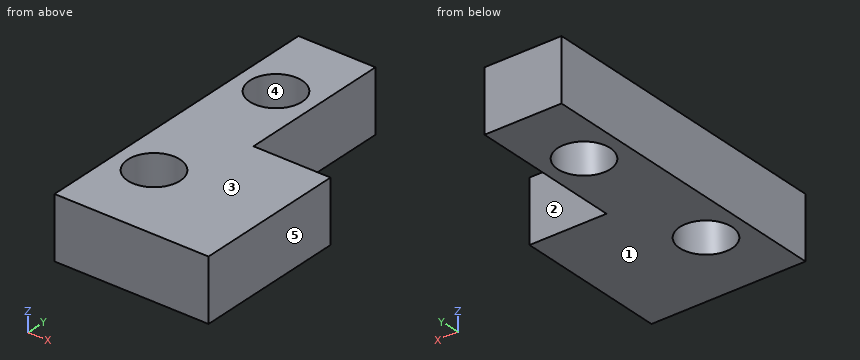
```python
from build123d import *

# Parameters (mm, degrees)
ESQUISSE1_W             = 10
ESQUISSE1_H             = 20
BOSS_EXTRU_1_DEPTH      = 4
D_GAGEMENT_M33_D        = 3.4
ESQUISSE2_W             = 5
ESQUISSE2_H             = 10
ENL_V_MAT_EXTRU_2_DEPTH = 4


with BuildPart() as part:
    # Esquisse1 → Boss.-Extru.1 (new body)
    with BuildSketch(Plane.XY):
        Rectangle(ESQUISSE1_W, ESQUISSE1_H)
    extrude(amount=BOSS_EXTRU_1_DEPTH)

    # Dégagement M33 (through all)
    with Locations(Plane(origin=(0, 0, 0), x_dir=(-1, 0, 0), z_dir=(0, 0, -1))):
        with Locations((2.5, 5), (2.5, -5)):
            Hole(D_GAGEMENT_M33_D / 2)

    # Esquisse2 → Enlèv. mat.-Extru.2 (cut)
    with BuildSketch(Plane(origin=(0, 0, 0), x_dir=(-1, 0, 0), z_dir=(0, 0, -1))):
        with Locations((-2.5, 5)):
            Rectangle(ESQUISSE2_W, ESQUISSE2_H)
    extrude(amount=-ENL_V_MAT_EXTRU_2_DEPTH, mode=Mode.SUBTRACT)


solid = part.part
```
The model under review builds one solid part; all positions refer to its coordinate system, in mm. Face numbers are marked on the shaded views. A direction names the side the tool comes from. Give positions to 0.01 mm unless a question says otherwise; leave off trailing zeros. Write each loop counter-clockwise with the first axis right and the second up, starting at its lowest first coordinate (ties: lowest second). Pieces come first, ordered by that corner, then holes. Notation, with made-up numbers: M 66,22 L 76,22 A28 ccw 76,52 Z; hole C 85,-16.5 d3. An arc over 180 degrees is marked long. Answer in a Markdown table with one row per item.
Item 1: Tool access review of the marked faces 1 and 2: name each direction out of +Z, -Z, +X, -X, +Y, -Y from which nothing blocks a thin tool from reaching the whole face with its end or side.
Check sheet entries:
| item | result |
|---|---|
| face 1 | -Z, +X, -X, +Y, -Y |
| face 2 | +Z, -Z, +X, +Y |
Item 2: For P1, Ø2, axis at y = 4.5, z = 2.5, coming from the +X side; P2, Ø2.5, axis at x = -2.5, y = -5, coming from the +Z side, all flat-tipped, find the tip position at first contact; note any pin that passes through.
Check sheet entries:
| item | result |
|---|---|
| P1 | x = 0 |
| P2 | through |
Item 3: Add section A-A on y = -5. Give the boundary of the cut face in (x, z), plus the area to 3 significant figures.
Check sheet entries:
| item | result |
|---|---|
| outline | M -5,0 L -4.2,0 L -4.2,4 L -5,4 Z; M -0.8,0 L 5,0 L 5,4 L -0.8,4 Z |
| area | 26.4 mm2 |
Item 4: Draft analysis for pull direction X (two halves, no side actions). For the marked faces 3, 4 and 5, state which applies: +X half, -X half, draft (parallel to the pull), parting line (faces both ways), or undercut.
Check sheet entries:
| item | result |
|---|---|
| face 3 | draft |
| face 4 | undercut |
| face 5 | +X half |
Item 5: For line 1 along Y through (x, z) = (-2.5, 3.25); line 2 along Y through (x, z) = (-3, 3); line 3 along Y through (x, z) = (1, 0.4), list the stretches that pass through material, from the lowest coordinate up.
Check sheet entries:
| item | result |
|---|---|
| line 1 | -10 to -6.7, -3.3 to 3.3, 6.7 to 10 |
| line 2 | -10 to -6.62, -3.38 to 3.38, 6.62 to 10 |
| line 3 | -10 to 0 |
Item 6: Add section D-D on y = 5. Give the boundary of the cut face in (x, z).
Check sheet entries:
| item | result |
|---|---|
| outline | M -5,0 L -4.2,0 L -4.2,4 L -5,4 Z; M -0.8,0 L 0,0 L 0,4 L -0.8,4 Z |
Item 7: Add section C-C on z = 2. Give the boundary of the cut face in (x, y).
Check sheet entries:
| item | result |
|---|---|
| outline | M -5,-10 L 5,-10 L 5,0 L 0,0 L 0,10 L -5,10 Z; hole C -2.5,-5 d3.4; hole C -2.5,5 d3.4 |
Item 8: Add section B-B on x = -2.5. Give the boundary of the cut face in (y, z).
Check sheet entries:
| item | result |
|---|---|
| outline | M -10,0 L -6.7,0 L -6.7,4 L -10,4 Z; M -3.3,0 L 3.3,0 L 3.3,4 L -3.3,4 Z; M 6.7,0 L 10,0 L 10,4 L 6.7,4 Z |
